from build123d import *

# Parameters (mm, degrees)
SKETCH1_W           = 200
SKETCH1_H           = 40
BOSS_EXTRUDE1_DEPTH = 3
SKETCH2_W           = 5
SKETCH2_H           = 200
BOSS_EXTRUDE2_DEPTH = 60
SKETCH4_R           = 4
CUT_EXTRUDE1_DEPTH  = 60
FILLET2_R           = 3


with BuildPart() as part:
    # Sketch1 → Boss-Extrude1 (new body)
    with BuildSketch(Plane(origin=(0, 0, 0), x_dir=(0, 1, 0), z_dir=(0, 0, 1))):
        Rectangle(SKETCH1_W, SKETCH1_H)
    extrude(amount=BOSS_EXTRUDE1_DEPTH)

    # Sketch2 → Boss-Extrude2 (add)
    with BuildSketch(Plane.XY.offset(3)):
        with Locations((-17.5, 0)):
            Rectangle(SKETCH2_W, SKETCH2_H)
        with Locations((17.5, 0)):
            Rectangle(SKETCH2_W, SKETCH2_H)
    extrude(amount=BOSS_EXTRUDE2_DEPTH)

    # Sketch4 → Cut-Extrude1 (cut)
    with BuildSketch(Plane(origin=(-20, 0, 0), x_dir=(0, -1, 0), z_dir=(-1, 0, 0))):
        with BuildLine():
            Line((-100, 63), (-100, 20))
            ThreePointArc((-100, 20), (-85, 35), (-70, 20))
            Line((-70, 20), (-15, 60))
            Line((-15, 60), (65, 60))
            Line((65, 60), (65, 0))
            Line((65, 0), (100, 0))
            Line((100, 0), (100, 63))
            Line((100, 63), (-100, 63))
        make_face()
        with Locations(Location((-85, 20, 0), (0, 0, 90))):
            Circle(SKETCH4_R)
        with Locations(Location((5, 45, 0), (0, 0, 90))):
            Circle(SKETCH4_R)
        with Locations(Location((46, 45, 0), (0, 0, 90))):
            Circle(SKETCH4_R)
    extrude(amount=-CUT_EXTRUDE1_DEPTH, mode=Mode.SUBTRACT)

    # Fillet2
    fillet2_edges = [part.edges().sort_by_distance(p)[0] for p in [
        (17.5, 70, 20),
        (-17.5, 70, 20),
        (17.5, 15, 60),
        (-17.5, 15, 60),
    ]]
    fillet(fillet2_edges, radius=FILLET2_R)


solid = part.part
Model file for the job. Use its own axes, mm. A direction names the side the tool comes from. Give positions to 0.01 mm unless a question says otherwise; leave off trailing zeros. Loops run counter-clockwise (first coordinate to the right, second up) from the corner with the lowest first, then second, coordinate; pieces in that order, holes last.
Item 1: Slice it at A-A (z = 8.5). Write the cut outline in (x, y), plus the area to 3 significant figures.
Check values:
outline: (-20, -65) - (-15, -65) - (-15, 100) - (-20, 100) - close; (15, -65) - (20, -65) - (20, 100) - (15, 100) - close
area: 1,650 mm2
Item 2: Slice it at B-B (y = 85). Write the cut outline in (x, z), plus the area to 3 significant figures.
Check values:
outline: (-20, 0) - (20, 0) - (20, 16) - (15, 16) - (15, 3) - (-15, 3) - (-15, 16) - (-20, 16) - close; (-20, 24) - (-15, 24) - (-15, 35) - (-20, 35) - close; (15, 24) - (20, 24) - (20, 35) - (15, 35) - close
area: 360 mm2
Item 3: Drop a flat-ended pin along its axis: P1, Ø15, axis at x = 6.5, y = 32, coming from the +Z side. Give the stop position or say it passes through.
Check values:
P1: stops at z = 3
Item 4: Mould opens along Y. For faces 1 (the face through (17.465, 87.532, 34.785)), 2 (the face through (-17.535, 87.532, 34.785)), 3 (the face through (-0.1, 100, 2.5)), 4 (the face through (-18, -25, 60)) say: +Y half, -Y half, draft (parallel to the pull), parting line (faces both ways), or undercut.
Check values:
face 1: undercut
face 2: undercut
face 3: +Y half
face 4: draft
Item 5: Which spindle directions (+Z, -Z, +X, -X, +Y, -Y) get a long thin tool onto all of the face, cutting with end or side? Do faces 5 (the face through (-20, -2, 23)), 6 (the face through (-17.54, 41.26, 40.9)), 7 (the face through (-15, -2, 25)). Say none if no direction does.
Check values:
face 5: +Z, -Z, -X, +Y, -Y
face 6: +Z, +X, -X
face 7: +Z, +Y, -Y
Item 6: Slice it at C-C (y = 4). Write the cut outline in (x, z).
Check values:
outline: (-20, 0) - (20, 0) - (20, 60) - (15, 60) - (15, 3) - (-15, 3) - (-15, 60) - (-20, 60) - close
Item 7: Drill centre lines: line 1 along X through (y, z) = (25, 22); line 2 along Y through (x, z) = (-18, 45) (3 decimals); line 3 along Y through (x, z) = (-17.5, 46). Where is each one in solid material? Low to high.
Check values:
line 1: x = -20 to -15, 15 to 20
line 2: y = -65 to -50, -42 to -9, -1 to 35.625
line 3: y = -65 to -49.87, -42.13 to -8.87, -1.13 to 34.25
Item 8: Slice it at D-D (z = 45). Write the cut outline in (x, y) (3 decimals), plus the area to 3 significant figures.
Check values:
outline: (-20, -65) - (-15, -65) - (-15, -50) - (-20, -50) - close; (-20, -42) - (-15, -42) - (-15, -9) - (-20, -9) - close; (-20, -1) - (-15, -1) - (-15, 35.625) - (-20, 35.625) - close; (15, -65) - (20, -65) - (20, -50) - (15, -50) - close; (15, -42) - (20, -42) - (20, -9) - (15, -9) - close; (15, -1) - (20, -1) - (20, 35.625) - (15, 35.625) - close
area: 846 mm2
